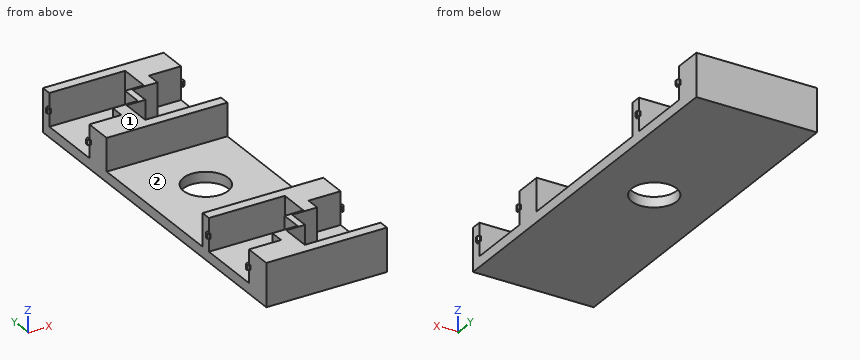
```python
from build123d import *

# Parameters (mm, degrees)
F0_R     = 6.5
F1_DEPTH = 3
F2_DEPTH = 9.5
F3_W     = 0.6965331137
F3_H     = 1.3967012055
F3_W_2   = 0.8034668863
F3_W_3   = 0.836771971
F3_W_4   = 0.663228029
F3_W_5   = 0.7633265793
F3_W_6   = 0.7366734207
F3_W_7   = 0.7139041424
F3_W_8   = 0.7860958576
F4_DEPTH = 0.75
F5_W     = 0.7277277052
F5_H     = 1.3967012055
F5_W_2   = 0.7722722948
F5_W_3   = 0.7690980434
F5_W_4   = 0.7309019566
F5_W_5   = 0.6904412746
F5_W_6   = 0.8095587254
F5_W_7   = 0.7503486574
F5_W_8   = 0.7496513426
F6_DEPTH = 0.75
F7_SIZE  = 0.5


# Not quite as in the source:
# - ends of sketch curves that miss each other by under 0.0002 mm in the source are joined
# - a feature names something its author has since deleted; it is built from what else it names


with BuildPart() as f1:
    # F0 (on Top) → F1 (new body)
    with BuildSketch(Plane.XY):
        Polygon((7.8607099131, 16.1003852367), (-9.6392899379, 16.1003852367), (-9.6392899379, -29.3996147633), (25.3607097641, -29.3996147633), (25.3607097641, 16.1003852367), align=None)
        with Locations((7.8607099131, -2.2867515218)):
            Circle(F0_R, mode=Mode.SUBTRACT)
        Polygon((25.3607097641, -29.3996147633), (-9.6392899379, -29.3996147633), (-9.6392899379, -32.3996147633), (-6.4715547308, -32.3996147633), (12.3607100621, -32.3996147633), (25.3607097641, -32.3996147633), align=None)
        Polygon((-9.6392899379, 46.3003852367), (-9.6392899379, 43.3003852367), (-6.4715547308, 43.3003852367), (12.3607100621, 43.3003852367), (25.3607097641, 43.3003852367), (25.3607097641, 46.3003852367), align=None)
        Polygon((16.0607097641, 38.1003852367), (25.3607097641, 38.1003852367), (25.3607097641, 43.3003852367), (12.3607100621, 43.3003852367), (12.3607100621, 35.3003852367), (12.3607100621, 34.5003852367), (7.8607097641, 34.5003852367), (7.8607100621, 33.9926332235), (8.7954637781, 33.9926332235), (16.0607097641, 33.9926332235), align=None)
        Polygon((-9.6392899379, 43.3003852367), (-9.6392899379, 24.3003852367), (-0.3392899379, 24.3003852367), (-0.3392899379, 28.4081372499), (6.9259563461, 28.4081372499), (6.9259563461, 34.5003852367), (7.8607100621, 34.5003852367), (12.3607100621, 34.5003852367), (12.3607100621, 35.3003852367), (12.3607100621, 43.3003852367), (-6.4715547308, 43.3003852367), align=None)
        Polygon((3.3607097641, 27.1003852367), (3.3607097641, 19.1003852367), (22.192974557, 19.1003852367), (25.3607097641, 19.1003852367), (25.3607097641, 38.1003852367), (16.0607097641, 38.1003852367), (16.0607097641, 33.9926332235), (8.7954637781, 33.9926332235), (8.7954637781, 27.9003852367), (7.8607100621, 27.9003852367), (3.3607097641, 27.9003852367), align=None)
        Polygon((-9.6392899379, 19.1003852367), (-9.6392899379, 16.1003852367), (7.8607099131, 16.1003852367), (25.3607097641, 16.1003852367), (25.3607097641, 19.1003852367), (22.192974557, 19.1003852367), (3.3607097641, 19.1003852367), align=None)
        Polygon((-9.6392899379, 24.3003852367), (-9.6392899379, 19.1003852367), (3.3607097641, 19.1003852367), (3.3607097641, 27.1003852367), (3.3607097641, 27.9003852367), (7.8607100621, 27.9003852367), (7.8607100621, 28.4081372499), (6.9259563461, 28.4081372499), (-0.3392899379, 28.4081372499), (-0.3392899379, 24.3003852367), align=None)
        Polygon((6.9259563461, 34.5003852367), (6.9259563461, 28.4081372499), (7.8607097641, 28.4081372499), (7.8607100621, 33.9926332235), (7.8607100621, 34.5003852367), align=None)
        Polygon((7.8607100621, 28.4081372499), (7.8607100621, 27.9003852367), (8.7954637781, 27.9003852367), (8.7954637781, 33.9926332235), (7.8607097641, 33.9926332235), align=None)
        Polygon((-6.4715547308, -32.3996147633), (-9.6392899379, -32.3996147633), (-9.6392899379, -51.3996147633), (-0.3392899379, -51.3996147633), (-0.3392899379, -47.2918627501), (6.9259563461, -47.2918627501), (6.9259563461, -41.1996147633), (7.8607100621, -41.1996147633), (12.3607100621, -41.1996147633), (12.3607100621, -40.3996147633), (12.3607100621, -32.3996147633), align=None)
        Polygon((25.3607097641, -56.5996147633), (25.3607097641, -37.5996147633), (16.0607097641, -37.5996147633), (16.0607097641, -41.7073667765), (8.7954637781, -41.7073667765), (8.7954637781, -47.7996147633), (7.8607100621, -47.7996147633), (3.3607097641, -47.7996147633), (3.3607097641, -48.5996147633), (3.3607097641, -56.5996147633), (22.192974557, -56.5996147633), align=None)
        Polygon((25.3607097641, -37.5996147633), (25.3607097641, -32.3996147633), (12.3607100621, -32.3996147633), (12.3607100621, -40.3996147633), (12.3607100621, -41.1996147633), (7.8607097641, -41.1996147633), (7.8607100621, -41.7073667765), (8.7954637781, -41.7073667765), (16.0607097641, -41.7073667765), (16.0607097641, -37.5996147633), align=None)
        Polygon((-0.3392899379, -51.3996147633), (-9.6392899379, -51.3996147633), (-9.6392899379, -56.5996147633), (3.3607097641, -56.5996147633), (3.3607097641, -48.5996147633), (3.3607097641, -47.7996147633), (7.8607100621, -47.7996147633), (7.8607100621, -47.2918627501), (6.9259563461, -47.2918627501), (-0.3392899379, -47.2918627501), align=None)
        Polygon((8.7954637781, -47.7996147633), (8.7954637781, -41.7073667765), (7.8607097641, -41.7073667765), (7.8607100621, -47.2918627501), (7.8607100621, -47.7996147633), align=None)
        Polygon((6.9259563461, -41.1996147633), (6.9259563461, -47.2918627501), (7.8607097641, -47.2918627501), (7.8607100621, -41.7073667765), (7.8607100621, -41.1996147633), align=None)
        Polygon((3.3607097641, -56.5996147633), (-9.6392899379, -56.5996147633), (-9.6392899379, -59.5996147633), (25.3607097641, -59.5996147633), (25.3607097641, -56.5996147633), (22.192974557, -56.5996147633), align=None)
    extrude(amount=-F1_DEPTH)

    # F0 (on Top) → F2 (join)
    with BuildSketch(Plane.XY):
        Polygon((-9.6392899379, 19.1003852367), (-9.6392899379, 16.1003852367), (7.8607099131, 16.1003852367), (25.3607097641, 16.1003852367), (25.3607097641, 19.1003852367), (22.192974557, 19.1003852367), (3.3607097641, 19.1003852367), align=None)
        Polygon((-9.6392899379, 24.3003852367), (-9.6392899379, 19.1003852367), (3.3607097641, 19.1003852367), (3.3607097641, 27.1003852367), (3.3607097641, 27.9003852367), (7.8607100621, 27.9003852367), (7.8607100621, 28.4081372499), (6.9259563461, 28.4081372499), (-0.3392899379, 28.4081372499), (-0.3392899379, 24.3003852367), align=None)
        Polygon((-9.6392899379, 46.3003852367), (-9.6392899379, 43.3003852367), (-6.4715547308, 43.3003852367), (12.3607100621, 43.3003852367), (25.3607097641, 43.3003852367), (25.3607097641, 46.3003852367), align=None)
        Polygon((16.0607097641, 38.1003852367), (25.3607097641, 38.1003852367), (25.3607097641, 43.3003852367), (12.3607100621, 43.3003852367), (12.3607100621, 35.3003852367), (12.3607100621, 34.5003852367), (7.8607097641, 34.5003852367), (7.8607100621, 33.9926332235), (8.7954637781, 33.9926332235), (16.0607097641, 33.9926332235), align=None)
        Polygon((6.9259563461, 34.5003852367), (6.9259563461, 28.4081372499), (7.8607097641, 28.4081372499), (7.8607100621, 33.9926332235), (7.8607100621, 34.5003852367), align=None)
        Polygon((7.8607100621, 28.4081372499), (7.8607100621, 27.9003852367), (8.7954637781, 27.9003852367), (8.7954637781, 33.9926332235), (7.8607097641, 33.9926332235), align=None)
        Polygon((25.3607097641, -29.3996147633), (-9.6392899379, -29.3996147633), (-9.6392899379, -32.3996147633), (-6.4715547308, -32.3996147633), (12.3607100621, -32.3996147633), (25.3607097641, -32.3996147633), align=None)
        Polygon((25.3607097641, -37.5996147633), (25.3607097641, -32.3996147633), (12.3607100621, -32.3996147633), (12.3607100621, -40.3996147633), (12.3607100621, -41.1996147633), (7.8607097641, -41.1996147633), (7.8607100621, -41.7073667765), (8.7954637781, -41.7073667765), (16.0607097641, -41.7073667765), (16.0607097641, -37.5996147633), align=None)
        Polygon((-0.3392899379, -51.3996147633), (-9.6392899379, -51.3996147633), (-9.6392899379, -56.5996147633), (3.3607097641, -56.5996147633), (3.3607097641, -48.5996147633), (3.3607097641, -47.7996147633), (7.8607100621, -47.7996147633), (7.8607100621, -47.2918627501), (6.9259563461, -47.2918627501), (-0.3392899379, -47.2918627501), align=None)
        Polygon((8.7954637781, -47.7996147633), (8.7954637781, -41.7073667765), (7.8607097641, -41.7073667765), (7.8607100621, -47.2918627501), (7.8607100621, -47.7996147633), align=None)
        Polygon((6.9259563461, -41.1996147633), (6.9259563461, -47.2918627501), (7.8607097641, -47.2918627501), (7.8607100621, -41.7073667765), (7.8607100621, -41.1996147633), align=None)
        Polygon((3.3607097641, -56.5996147633), (-9.6392899379, -56.5996147633), (-9.6392899379, -59.5996147633), (25.3607097641, -59.5996147633), (25.3607097641, -56.5996147633), (22.192974557, -56.5996147633), align=None)
    extrude(amount=F2_DEPTH)

    # F3 (on face) → F4 (join)
    with BuildSketch(Plane.YZ.offset(25.3607097641)):
        with Locations((19.4486517936, 4.715041643)):
            Rectangle(F3_W, F3_H)
        with Locations((18.6986517936, 4.715041643)):
            Rectangle(F3_W_2, F3_H)
        with Locations((37.6819992512, 4.7070782166)):
            Rectangle(F3_W_3, F3_H)
        with Locations((38.4319992512, 4.7070782166)):
            Rectangle(F3_W_4, F3_H)
        with Locations((-37.2179514736, 4.7070782166)):
            Rectangle(F3_W_5, F3_H)
        with Locations((-37.9679514736, 4.7070782166)):
            Rectangle(F3_W_6, F3_H)
        with Locations((-56.2426626921, 4.715041643)):
            Rectangle(F3_W_7, F3_H)
        with Locations((-56.9926626921, 4.715041643)):
            Rectangle(F3_W_8, F3_H)
    extrude(amount=F4_DEPTH)

    # F5 (on face) → F6 (join)
    with BuildSketch(Plane(origin=(-9.6392899379, 0, 0), x_dir=(0, -1, 0), z_dir=(-1, 0, 0))):
        with Locations((51.7634786159, 4.7070782166)):
            Rectangle(F5_W, F5_H)
        with Locations((51.0134786159, 4.7070782166)):
            Rectangle(F5_W_2, F5_H)
        with Locations((32.784163785, 4.715041643)):
            Rectangle(F5_W_3, F5_H)
        with Locations((32.034163785, 4.715041643)):
            Rectangle(F5_W_4, F5_H)
        with Locations((-23.9551645994, 4.7070782166)):
            Rectangle(F5_W_5, F5_H)
        with Locations((-24.7051645994, 4.7070782166)):
            Rectangle(F5_W_6, F5_H)
        with Locations((-42.9252109081, 4.715041643)):
            Rectangle(F5_W_7, F5_H)
        with Locations((-43.6752109081, 4.715041643)):
            Rectangle(F5_W_8, F5_H)
    extrude(amount=F6_DEPTH)

    # F7
    f7_edges = [f1.edges().sort_by_distance(p)[0] for p in [
        (26.11071, 38.763613, 4.707078),
        (26.11071, 37.263613, 4.707078),
        (26.11071, 19.796918, 4.715042),
        (26.11071, 18.296918, 4.715042),
        (26.11071, -36.836288, 4.707078),
        (26.11071, -38.336288, 4.707078),
        (26.11071, -55.885711, 4.715042),
        (26.11071, -57.385711, 4.715042),
        (-10.38929, -52.127342, 4.707078),
        (-10.38929, -50.627342, 4.707078),
        (-10.38929, -33.168713, 4.715042),
        (-10.38929, -31.668713, 4.715042),
        (-10.38929, 23.609944, 4.707078),
        (-10.38929, 25.109944, 4.707078),
        (-10.38929, 42.550037, 4.715042),
        (-10.38929, 44.050037, 4.715042),
    ]]
    chamfer(f7_edges, length=F7_SIZE)


solid = f1.part
```
Geometry: final body of the model. Coordinates: model frame, mm. Face numbers are marked on the shaded views. A direction names the side the tool comes from. Coordinates: 2 decimals unless noted, no trailing zeros. Order: outer loops, then holes, each group sorted by start corner. A loop starts at its lowest first (then second) coordinate and runs counter-clockwise, first axis right, second up. Notation, with made-up numbers: M 1.5,75.5 L 51.5,75.5 A30 cw 51.5,98.5 Z; hole C -5,-14 d8. An arc over 180 degrees is marked long. Answer in a Markdown table with one row per item. Add a question column.
Q1. Contact query for flat-ended pins moving along their axis: P1, Ø2.5, axis at y = 40, z = 5, coming from the -X side; P2, Ø3, axis at y = 11, z = -1.5, coming from the -X side; P3, Ø3, axis at x = -0.5, y = -12.5, coming from the +Z side. Output: stop coordinate, or through.
Q2. Section query C-C on x = 10. Return the cut outline in (y, z).
Q3. Reachability of the marked faces 1 and 2 from +Z, -Z, +X, -X, +Y, -Y: full face, straight path, thin tool, end or side. Return the list, or none.
Q4. Section query B-B on x = -5. Return the cut outline in (y, z), and give its area (4 significant figures).
Q5. Section query A-A on y = -4. Return the cut outline in (x, z).
Q6. Line query: L1, parallel to Y at x = 14, z = 7; L2, parallel to Y at x = 11, z = 7.5; L3, parallel to Y at x = 17.5, z = 3.75. Output: solid intervals per line, ascending.
Q7. Section query D-D on z = -2. Return the cut outline in (x, y), and give its area (3 significant figures).
Completed:
| question | item | result |
|---|---|---|
| 1 | P1 | stops at x = 12.36 |
| 1 | P2 | stops at x = -9.64 |
| 1 | P3 | stops at z = 0 |
| 2 | outline | M -59.6,-3 L -8.42,-3 L -8.42,0 L -29.4,0 L -29.4,9.5 L -32.4,9.5 L -32.4,0 L -41.2,0 L -41.2,9.5 L -41.71,9.5 L -41.71,0 L -56.6,0 L -56.6,9.5 L -59.6,9.5 Z; M 3.85,-3 L 46.3,-3 L 46.3,9.5 L 43.3,9.5 L 43.3,0 L 34.5,0 L 34.5,9.5 L 33.99,9.5 L 33.99,0 L 19.1,0 L 19.1,9.5 L 16.1,9.5 L 16.1,0 L 3.85,0 Z |
| 3 | face 1 | +Z, +X, -X, +Y, -Y |
| 3 | face 2 | +Z, +X, -X |
| 4 | outline | M -59.6,-3 L 46.3,-3 L 46.3,9.5 L 43.3,9.5 L 43.3,0 L 24.3,0 L 24.3,9.5 L 16.1,9.5 L 16.1,0 L -29.4,0 L -29.4,9.5 L -32.4,9.5 L -32.4,0 L -51.4,0 L -51.4,9.5 L -59.6,9.5 Z |
| 4 | area | 530.5 mm2 |
| 5 | outline | M -9.64,-3 L 1.59,-3 L 1.59,0 L -9.64,0 Z; M 14.13,-3 L 25.36,-3 L 25.36,0 L 14.13,0 Z |
| 6 | L1 | y = -59.6 to -56.6, -41.71 to -29.4, 16.1 to 19.1, 33.99 to 46.3 |
| 6 | L2 | y = -59.6 to -56.6, -41.71 to -41.2, -32.4 to -29.4, 16.1 to 19.1, 33.99 to 34.5, 43.3 to 46.3 |
| 6 | L3 | y = -59.6 to -56.6, -37.6 to -29.4, 16.1 to 19.1, 38.1 to 46.3 |
| 7 | outline | M -9.64,-59.6 L 25.36,-59.6 L 25.36,46.3 L -9.64,46.3 Z; hole C 7.86,-2.29 d13 |
| 7 | area | 3,570 mm2 |
